Here's how the part is built. I have some questions about the finished solid (model axes, mm). Face numbers are marked on the shaded views. A direction names the side the tool comes from. Coordinates: 2 decimals unless noted, no trailing zeros. Write each loop counter-clockwise with the first axis right and the second up, starting at its lowest first coordinate (ties: lowest second). Pieces come first, ordered by that corner, then holes.
(1) For pin 1 Ø4 at (x, y) = (2, 28.5) entering from +Z (3 decimals); pin 2 Ø1.5 at (y, z) = (25.5, 0.5) entering from -X (3 decimals); pin 3 Ø6 at (y, z) = (46, -0.5) entering from +X (3 decimals), each with a flat end and sliding along its axis, tell me the tip position at first contact or that it passes through.
(2) Imagine slicing it at C-C, the plane z = 0. List the corners of the cut face in (x, y) for me (3 decimals), plus the area to 3 significant figures.
(3) Imagine slicing it at A-A, the plane y = 6. List the corners of the cut face in (x, z) for me (3 decimals), plus the area to 3 significant figures.
(4) Which directions (+Z, -Z, +X, -X, +Y, -Y) give clear straight access to the entire face, cutting with the end or side of a thin tool? Please do the marked faces 1 and 2.
(5) Imagine slicing it at D-D, the plane z = -4. List the corners of the cut face in (x, y) for me, plus the area to 3 significant figures.
(6) Imagine slicing it at B-B, the plane x = 0. List the corners of the cut face in (y, z) for me (3 decimals).
(7) Please list where these lines run through material, in increasing order: probe 1 along Y at (x, z) = (-2.75, -5.25); probe 2 along X at (y, z) = (45, -0.25); probe 3 along X at (y, z) = (31.5, -1.5).
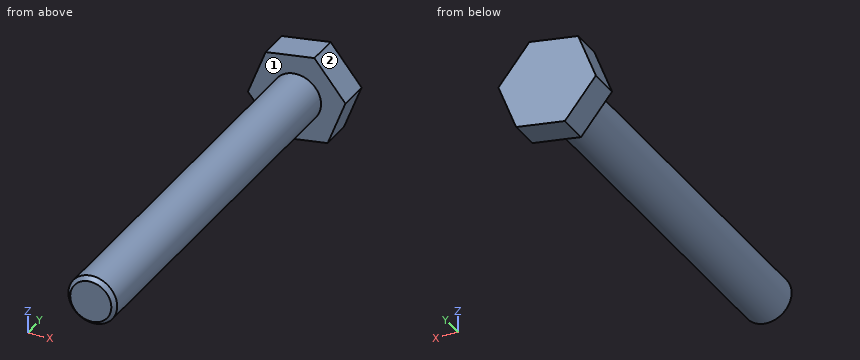
```python
from build123d import *

# Parameters (mm, degrees)
SKETCH1_R           = 3.175
BOSS_EXTRUDE1_DEPTH = 50.8
BOSS_EXTRUDE2_DEPTH = 4
CHAMFER1_SIZE       = 0.5


with BuildPart() as part:
    # Sketch1 → Boss-Extrude1 (new body)
    with BuildSketch(Plane(origin=(0, 0, 0), x_dir=(1, 0, 0), z_dir=(0, 1, 0))):
        with Locations(Location((0, 0, 0), (0, 0, 270))):
            Circle(SKETCH1_R)
    extrude(amount=BOSS_EXTRUDE1_DEPTH)

    # Sketch2 → Boss-Extrude2 (add)
    with BuildSketch(Plane(origin=(0, 50.8, 0), x_dir=(1, 0, 0), z_dir=(0, 1, 0))):
        Polygon((-2.30492787, 5.987475227), (-6.337769586, 0.997611524), (-4.032841716, -4.989863703), (2.30492787, -5.987475227), (6.337769586, -0.997611524), (4.032841716, 4.989863703), align=None)
    extrude(amount=BOSS_EXTRUDE2_DEPTH)

    # Chamfer1
    chamfer1_edges = [part.edges().sort_by_distance(p)[0] for p in [
        (0, 0, -3.175),
    ]]
    chamfer(chamfer1_edges, length=CHAMFER1_SIZE)


solid = part.part
```
Recorded:
1. pin 1: stops at z = 3.175
1. pin 2: stops at x = -3.175
1. pin 3: stops at x = 3.175
2. outline: (-5.954, 50.8) - (-3.175, 50.8) - (-3.175, 0.5) - (-2.675, 0) - (2.675, 0) - (3.175, 0.5) - (3.175, 50.8) - (5.954, 50.8) - (5.954, 54.8) - (-5.954, 54.8) - close
2. area: 370 mm2
3. outline: circle Ø6.35 at (0, 0)
3. area: 31.7 mm2
4. face 1: -Y
4. face 2: +Z, +X, +Y, -Y
5. outline: (-3.91, 50.8) - (4.41, 50.8) - (4.41, 54.8) - (-3.91, 54.8) - close
5. area: 33.3 mm2
6. outline: (0, -2.675) - (0.5, -3.175) - (50.8, -3.175) - (50.8, -5.625) - (54.8, -5.625) - (54.8, 5.625) - (50.8, 5.625) - (50.8, 3.175) - (0.5, 3.175) - (0, 2.675) - close
7. probe 1: y = 50.8 to 54.8
7. probe 2: x = -3.17 to 3.17
7. probe 3: x = -2.8 to 2.8
